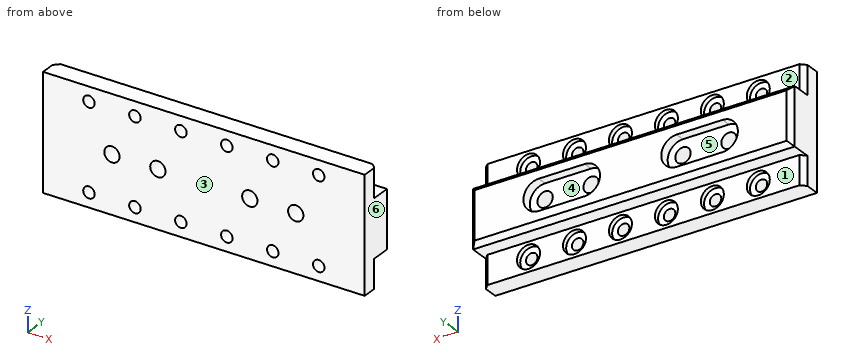
from build123d import *

# Parameters (mm, degrees)
BOSS_EXTRUDE1_DEPTH = 106.68
SKETCH3_R           = 3.81
CUT_EXTRUDE1_DEPTH  = 114.989132815
SKETCH5_R           = 7.62
CUT_EXTRUDE2_DEPTH  = 3.175
SKETCH6_R           = 5.08
CUT_EXTRUDE3_DEPTH  = 117.092172001
CUT_EXTRUDE4_DEPTH  = 6.35
CHAMFER1_SIZE       = 3.175


with BuildPart() as part:
    # Sketch1 → Boss-Extrude1 (new, symmetric)
    with BuildSketch(Plane(origin=(0, 0, 0), x_dir=(0, 0, -1), z_dir=(1, 0, 0))):
        Polygon((38.1, 0), (-38.1, 0), (-38.1, 12.7), (-19.05, 12.7), (-19.05, 25.4), (19.05, 25.4), (19.05, 12.7), (38.1, 12.7), align=None)
    extrude(amount=BOSS_EXTRUDE1_DEPTH, both=True)

    # Sketch3 → Cut-Extrude1 (cut, through all)
    with BuildSketch(Plane(origin=(0, 12.7, 0), x_dir=(1, 0, 0), z_dir=(0, 1, 0))):
        with Locations(Location((-76.2, -28.575, 0), (0, 0, 270))):
            Circle(SKETCH3_R)
        with Locations(Location((-45.72, -28.575, 0), (0, 0, 270))):
            Circle(SKETCH3_R)
        with Locations(Location((-15.24, -28.575, 0), (0, 0, 270))):
            Circle(SKETCH3_R)
        with Locations(Location((15.24, -28.575, 0), (0, 0, 270))):
            Circle(SKETCH3_R)
        with Locations(Location((45.72, -28.575, 0), (0, 0, 270))):
            Circle(SKETCH3_R)
        with Locations(Location((76.2, -28.575, 0), (0, 0, 270))):
            Circle(SKETCH3_R)
        with Locations(Location((76.2, 28.575, 0), (0, 0, 90))):
            Circle(SKETCH3_R)
        with Locations(Location((45.72, 28.575, 0), (0, 0, 90))):
            Circle(SKETCH3_R)
        with Locations(Location((15.24, 28.575, 0), (0, 0, 90))):
            Circle(SKETCH3_R)
        with Locations(Location((-15.24, 28.575, 0), (0, 0, 90))):
            Circle(SKETCH3_R)
        with Locations(Location((-45.72, 28.575, 0), (0, 0, 90))):
            Circle(SKETCH3_R)
        with Locations(Location((-76.2, 28.575, 0), (0, 0, 90))):
            Circle(SKETCH3_R)
    extrude(amount=-CUT_EXTRUDE1_DEPTH, mode=Mode.SUBTRACT)

    # Sketch5 → Cut-Extrude2 (cut)
    with BuildSketch(Plane(origin=(0, 12.7, 0), x_dir=(1, 0, 0), z_dir=(0, 1, 0))):
        with Locations(Location((-76.2, -28.575, 0), (0, 0, 270))):
            Circle(SKETCH5_R)
        with Locations(Location((-45.72, -28.575, 0), (0, 0, 270))):
            Circle(SKETCH5_R)
        with Locations(Location((-15.24, -28.575, 0), (0, 0, 270))):
            Circle(SKETCH5_R)
        with Locations(Location((15.24, -28.575, 0), (0, 0, 270))):
            Circle(SKETCH5_R)
        with Locations(Location((45.72, -28.575, 0), (0, 0, 270))):
            Circle(SKETCH5_R)
        with Locations(Location((76.2, -28.575, 0), (0, 0, 270))):
            Circle(SKETCH5_R)
        with Locations(Location((-45.72, 28.575, 0), (0, 0, 270))):
            Circle(SKETCH5_R)
        with Locations(Location((-15.24, 28.575, 0), (0, 0, 270))):
            Circle(SKETCH5_R)
        with Locations(Location((15.24, 28.575, 0), (0, 0, 270))):
            Circle(SKETCH5_R)
        with Locations(Location((45.72, 28.575, 0), (0, 0, 270))):
            Circle(SKETCH5_R)
        with Locations(Location((76.2, 28.575, 0), (0, 0, 270))):
            Circle(SKETCH5_R)
        with Locations(Location((-76.2, 28.575, 0), (0, 0, 270))):
            Circle(SKETCH5_R)
    extrude(amount=-CUT_EXTRUDE2_DEPTH, mode=Mode.SUBTRACT)

    # Sketch6 → Cut-Extrude3 (cut, through all)
    with BuildSketch(Plane(origin=(0, 25.4, 0), x_dir=(1, 0, 0), z_dir=(0, 1, 0))):
        with Locations(Location((-60.96, 0, 0), (0, 0, 270))):
            Circle(SKETCH6_R)
        with Locations(Location((-30.48, 0, 0), (0, 0, 270))):
            Circle(SKETCH6_R)
        with Locations(Location((30.48, 0, 0), (0, 0, 90))):
            Circle(SKETCH6_R)
        with Locations(Location((60.96, 0, 0), (0, 0, 90))):
            Circle(SKETCH6_R)
    extrude(amount=-CUT_EXTRUDE3_DEPTH, mode=Mode.SUBTRACT)

    # Sketch7 → Cut-Extrude4 (cut)
    with BuildSketch(Plane(origin=(0, 25.4, 0), x_dir=(1, 0, 0), z_dir=(0, 1, 0))):
        with BuildLine():
            Line((-60.96, 10.16), (-30.48, 10.16))
            ThreePointArc((-30.48, 10.16), (-20.32, 0), (-30.48, -10.16))
            Line((-30.48, -10.16), (-60.96, -10.16))
            ThreePointArc((-60.96, -10.16), (-71.12, 0), (-60.96, 10.16))
        make_face()
        with BuildLine():
            Line((30.48, 10.16), (60.96, 10.16))
            ThreePointArc((60.96, 10.16), (71.12, 0), (60.96, -10.16))
            Line((60.96, -10.16), (30.48, -10.16))
            ThreePointArc((30.48, -10.16), (20.32, 0), (30.48, 10.16))
        make_face()
    extrude(amount=-CUT_EXTRUDE4_DEPTH, mode=Mode.SUBTRACT)

    # Chamfer1
    chamfer1_edges = [part.edges().sort_by_distance(p)[0] for p in [
        (-106.68, 25.4, 0),
        (-106.68, 12.7, -28.575),
        (106.68, 25.4, 0),
        (0, 25.4, 19.05),
        (0, 25.4, -19.05),
        (106.68, 12.7, 28.575),
        (106.68, 12.7, -28.575),
        (-106.68, 12.7, 28.575),
    ]]
    chamfer(chamfer1_edges, length=CHAMFER1_SIZE)


solid = part.part
The model under review builds one solid part; all positions refer to its coordinate system, in mm. Face numbers are marked on the shaded views. A direction names the side the tool comes from. Round coordinates to 2 decimals unless told otherwise and drop trailing zeros. Order: outer loops, then holes, each group sorted by start corner. A loop starts at its lowest first (then second) coordinate and runs counter-clockwise, first axis right, second up. Notation, with made-up numbers: (18, 28.25) -> (43, 28.25) arc R15 cw to (43, 33.25) -> close; hole circle Ø6 at (-25, 74). An arc over 180 degrees is marked (long way). Write item = value, one per line. Start each with the question number.
Item 1: For line 1 along X through (y, z) = (15.25, 0); line 2 along X through (y, z) = (24.25, -8.5) (3 decimals); line 3 along Y through (x, z) = (7, -29.5), list the stretches that pass through material, from the lowest coordinate up.
Item 2: Consider section D-D on x = -76.2. Write out the cut boundary in (y, z) (3 decimals).
Item 3: Clearance check with flat-ended pins moving along their axes: pin 1 Ø5 at (x, y) = (-19, 22.5) entering from -Z; pin 2 Ø7 at (x, y) = (-44.5, 22.5) entering from +Z; pin 3 Ø7.5 at (x, z) = (-43.5, -28.5) entering from +Y (3 decimals); pin 4 Ø8 at (x, z) = (-60.96, 0) entering from +Y. State where each tip first meets the part, or that it passes through.
Item 4: Consider section A-A on x = 45.72. Count the separate pieces of the cut face and the enclosed holes in it, plus the area to 3 significant figures.
Item 5: Mouldability with a two-part tool opening along Z and no side actions: class the marked faces 4, 5 and 6 as released by +Z, released by -Z, zero draft, split by the parting line, or undercut.
Item 6: For the marked faces 1, 2 and 3, list the 3-axis set-ups (+Z, -Z, +X, -X, +Y, -Y) from which the entire face can be reached by the end or side of a thin tool; tool diameter is ignored.
Conclusion:
q1.line_1 = -106.68 to -66.04, -55.88 to -35.56, -25.4 to 25.4, 35.56 to 55.88, 66.04 to 106.68
q1.line_2 = -104.655 to -66.526, -24.914 to 24.914, 66.526 to 104.655
q1.line_3 = 0 to 12.7
q2.outline = (0, -38.1) -> (12.7, -38.1) -> (12.7, -36.195) -> (9.525, -36.195) -> (9.525, -32.385) -> (0, -32.385) -> close; (0, -24.765) -> (9.525, -24.765) -> (9.525, -20.955) -> (12.7, -20.955) -> (12.7, -19.05) -> (22.225, -19.05) -> (25.4, -15.875) -> (25.4, 15.875) -> (22.225, 19.05) -> (12.7, 19.05) -> (12.7, 20.955) -> (9.525, 20.955) -> (9.525, 24.765) -> (0, 24.765) -> close; (0, 32.385) -> (9.525, 32.385) -> (9.525, 36.195) -> (12.7, 36.195) -> (12.7, 38.1) -> (0, 38.1) -> close
q3.pin_1 = -19.05
q3.pin_2 = 19.05
q3.pin_3 = 9.525
q3.pin_4 = through
q4.separate_pieces = 3
q4.enclosed_holes = 0
q4.area = 1,070 mm2
q5.face_4 = undercut
q5.face_5 = undercut
q5.face_6 = zero draft
q6.face_1 = -Z, +X, -X, +Y
q6.face_2 = +Z, +X, -X, +Y
q6.face_3 = +Z, -Z, +X, -X, -Y
